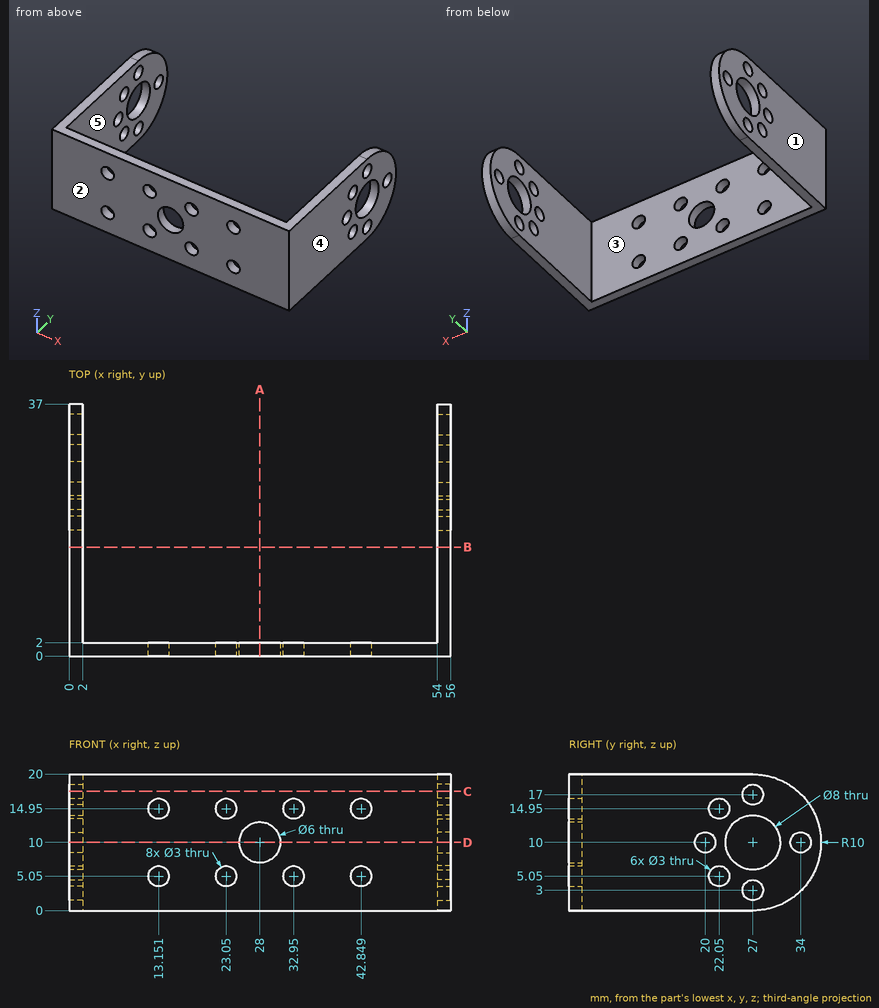
Design review of the part shown in the three views and the two pictorial views. Dimensions are in mm from the part's minimum x, y and z. A direction names the side the tool comes from. Coordinates: 2 decimals unless noted, no trailing zeros. Order: outer loops, then holes, each group sorted by start corner. A loop starts at its lowest first (then second) coordinate and runs counter-clockwise, first axis right, second up.
Item 1: Take a section at B-B, the plane y = 16. Write out the cut boundary in (x, z), then the cut area to 3 significant figures.
Item 2: For line 1 (X direction, y = 5, z = 6.5); line 2 (Y direction, x = 1.65, z = 10); line 3 (Y direction, x = 40, z = 7), list the stretches that pass through material, from the lowest coordinate up.
Item 3: For pin 1 Ø5 at (x, z) = (23.05, 5.05) entering from +Y; pin 2 Ø2.5 at (y, z) = (22.05, 14.95) entering from +X; pin 3 Ø4 at (y, z) = (27, 17) entering from -X, all flat-tipped, find the tip position at first contact; note any pin that passes through.
Item 4: The part is to be moulded in two halves that separate along X. For the marked faces 1, 2 and 3, say which applies: pulls with the +X half, pulls with the -X half, needs draft (parallel to the pull), parting line crosses it, or undercut.
Item 5: Take a section at C-C, the plane z = 17.5. Write out the cut boundary in (x, y).
Item 6: Take a section at A-A, the plane x = 28. Write out the cut boundary in (y, z), then the cut area to 3 significant figures.
Item 7: For the marked faces 4 and 5, list the 3-axis set-ups (+Z, -Z, +X, -X, +Y, -Y) from which the entire face can be reached by the end or side of a thin tool; tool diameter is ignored.
Item 8: Take a section at D-D, the plane z = 10. Count the separate pieces of the cut face and the enclosed holes in it, then the cut area to 3 significant figures.
The answers:
1. outline: (0, 0) - (2, 0) - (2, 20) - (0, 20) - close; (54, 0) - (56, 0) - (56, 20) - (54, 20) - close
1. area: 80.0 mm2
2. line 1: x = 0 to 2, 54 to 56
2. line 2: y = 0 to 18.5, 21.5 to 23, 31 to 32.5, 35.5 to 37
2. line 3: y = 0 to 2
3. pin 1: stops at y = 2
3. pin 2: passes through
3. pin 3: stops at x = 0
4. face 1: pulls with the -X half
4. face 2: needs draft
4. face 3: undercut
5. outline: (0, 0) - (56, 0) - (56, 25.59) - (54, 25.59) - (54, 2) - (2, 2) - (2, 25.59) - (0, 25.59) - close; (0, 28.41) - (2, 28.41) - (2, 33.61) - (0, 33.61) - close; (54, 28.41) - (56, 28.41) - (56, 33.61) - (54, 33.61) - close
6. outline: (0, 0) - (2, 0) - (2, 7) - (0, 7) - close; (0, 13) - (2, 13) - (2, 20) - (0, 20) - close
6. area: 28.0 mm2
7. face 4: +Z, -Z, +X, +Y, -Y
7. face 5: +Z, -Z, +Y
8. separate pieces: 8
8. enclosed holes: 0
8. area: 184 mm2
